The listing builds one solid part. Answer for the finished solid, in the listing's coordinates (mm). Face numbers are marked on the shaded views. A direction names the side the tool comes from. Coordinates: 2 decimals unless noted, no trailing zeros. Order: outer loops, then holes, each group sorted by start corner. A loop starts at its lowest first (then second) coordinate and runs counter-clockwise, first axis right, second up.
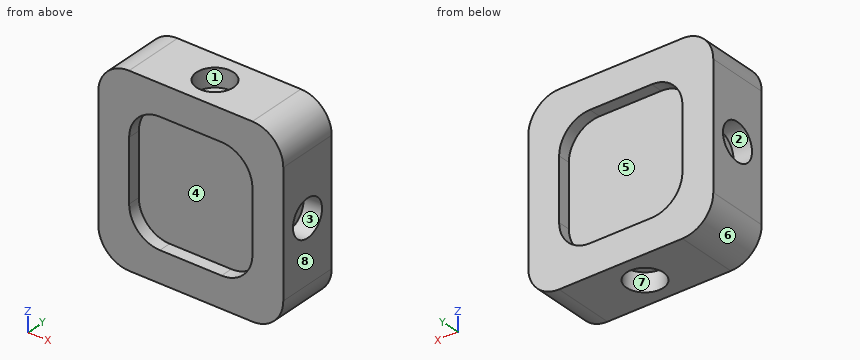
from build123d import *

# Parameters (mm, degrees)
SKETCH2_W           = 30
SKETCH2_H           = 30
BOSS_EXTRUDE1_DEPTH = 10
SKETCH3_R           = 3
CUT_EXTRUDE1_DEPTH  = 3
SKETCH4_R           = 3
CUT_EXTRUDE2_DEPTH  = 3
CUT_EXTRUDE3_START  = -3
SKETCH5_R           = 3
CUT_EXTRUDE3_DEPTH  = 3
CUT_EXTRUDE4_START  = -3
SKETCH6_R           = 3
CUT_EXTRUDE4_DEPTH  = 3
FILLET1_R           = 5
SKETCH8_W           = 20
SKETCH8_H           = 20
CUT_EXTRUDE6_DEPTH  = 2
FILLET2_R           = 5
SKETCH9_W           = 20
SKETCH9_H           = 20
CUT_EXTRUDE7_DEPTH  = 2
FILLET3_R           = 5


with BuildPart() as part:
    # Sketch2 → Boss-Extrude1 (new body)
    with BuildSketch(Plane(origin=(0, 0, 0), x_dir=(1, 0, 0), z_dir=(0, 1, 0))):
        Rectangle(SKETCH2_W, SKETCH2_H)
    extrude(amount=BOSS_EXTRUDE1_DEPTH)

    # Sketch3 → Cut-Extrude1 (cut)
    with BuildSketch(Plane.XY.offset(15)):
        with Locations((0, 5)):
            Circle(SKETCH3_R)
    extrude(amount=-CUT_EXTRUDE1_DEPTH, mode=Mode.SUBTRACT)

    # Sketch4 → Cut-Extrude2 (cut)
    with BuildSketch(Plane(origin=(15, 0, 0), x_dir=(0, 0, -1), z_dir=(1, 0, 0))):
        with Locations((0, 5)):
            Circle(SKETCH4_R)
    extrude(amount=-CUT_EXTRUDE2_DEPTH, mode=Mode.SUBTRACT)

    # Sketch5 → Cut-Extrude3 (cut)
    with BuildSketch(Plane(origin=(0, 0, -15), x_dir=(-1, 0, 0), z_dir=(0, 0, -1)).offset(CUT_EXTRUDE3_START)):
        with Locations(Location((0, 5, 0), (0, 0, 180))):
            Circle(SKETCH5_R)
    extrude(amount=CUT_EXTRUDE3_DEPTH, mode=Mode.SUBTRACT)

    # Sketch6 → Cut-Extrude4 (cut)
    with BuildSketch(Plane.ZY.offset(15).offset(CUT_EXTRUDE4_START)):
        with Locations(Location((0, 5, 0), (0, 0, 180))):
            Circle(SKETCH6_R)
    extrude(amount=CUT_EXTRUDE4_DEPTH, mode=Mode.SUBTRACT)

    # Fillet1
    fillet1_edges = [part.edges().sort_by_distance(p)[0] for p in [
        (15, 5, 15),
        (-15, 5, 15),
        (-15, 5, -15),
        (15, 5, -15),
    ]]
    fillet(fillet1_edges, radius=FILLET1_R)

    # Sketch8 → Cut-Extrude6 (cut)
    with BuildSketch(Plane(origin=(0, 10, 0), x_dir=(1, 0, 0), z_dir=(0, 1, 0))):
        Rectangle(SKETCH8_W, SKETCH8_H)
    extrude(amount=-CUT_EXTRUDE6_DEPTH, mode=Mode.SUBTRACT)

    # Fillet2
    fillet2_edges = [part.edges().sort_by_distance(p)[0] for p in [
        (10, 9, -10),
        (10, 9, 10),
        (-10, 9, 10),
        (-10, 9, -10),
    ]]
    fillet(fillet2_edges, radius=FILLET2_R)

    # Sketch9 → Cut-Extrude7 (cut)
    with BuildSketch(Plane(origin=(0, 0, 0), x_dir=(-1, 0, 0), z_dir=(0, -1, 0))):
        Rectangle(SKETCH9_W, SKETCH9_H)
    extrude(amount=-CUT_EXTRUDE7_DEPTH, mode=Mode.SUBTRACT)

    # Fillet3
    fillet3_edges = [part.edges().sort_by_distance(p)[0] for p in [
        (10, 1, 10),
        (10, 1, -10),
        (-10, 1, -10),
        (-10, 1, 10),
    ]]
    fillet(fillet3_edges, radius=FILLET3_R)


solid = part.part
1) Determine the mould class of the marked faces 5, 6, 7 and 8 for opening direction X: released by +X, released by -X, zero draft, split by the parting line, or undercut.
2) A tool of negligible diameter and unlimited length cuts with its end or side. For the marked faces 1, 2, 3 and 4, from which of +Z, -Z, +X, -X, +Y, -Y can it reach the whole face along a straight path? Write none if from no direction.
3) Section C-C (x = -5.75) is taken. Give the vertices of the cut face in (y, z), then the cut area to 3 significant figures.
4) Consider L1, parallel to Y at x = 0, z = -12.9; L2, parallel to Z at x = 0.25, y = 9; L3, parallel to Z at x = 1.5, y = 3. Determine where each line is inside the solid, lowest interval first.
5) Section D-D (x = -12.5) is taken. Give the vertices of the cut face in (y, z).
6) Section B-B (y = 5) is taken. Give the vertices of the cut face in (x, z), then the cut area to 3 significant figures.
7) Each of these flat-tipped pins is pushed along its axis until it touches: P1, Ø10, axis at x = -1.5, z = -3.5, coming from the +Y side; P2, Ø3.5, axis at x = 0, y = 5, coming from the -Z side; P3, Ø16, axis at x = 1.5, z = 1.5, coming from the -Y side. Where does it stop, or does it pass through?
8) Section A-A (z = 0) is taken. Give the vertices of the cut face in (x, y).
Filled sheet:
1. face 5: undercut
1. face 6: released by -X
1. face 7: undercut
1. face 8: released by +X
2. face 1: +Z
2. face 2: -X
2. face 3: +X
2. face 4: -Y
3. outline: (0, -15) - (10, -15) - (10, -9.94) - (8, -9.94) - (8, 9.94) - (10, 9.94) - (10, 15) - (0, 15) - (0, 9.94) - (2, 9.94) - (2, -9.94) - (0, -9.94) - close
3. area: 220 mm2
4. L1: y = 0 to 2, 8 to 10
4. L2: z = -15 to -10, 10 to 15
4. L3: z = -12 to 12
5. outline: (0, -14.33) - (10, -14.33) - (10, 14.33) - (0, 14.33) - close; hole circle Ø6 at (5, 0)
6. outline: (-15, -10) arc R5 ccw to (-10, -15) - (-3, -15) - (-3, -12) - (3, -12) - (3, -15) - (10, -15) arc R5 ccw to (15, -10) - (15, -3) - (12, -3) - (12, 3) - (15, 3) - (15, 10) arc R5 ccw to (10, 15) - (3, 15) - (3, 12) - (-3, 12) - (-3, 15) - (-10, 15) arc R5 ccw to (-15, 10) - (-15, 3) - (-12, 3) - (-12, -3) - (-15, -3) - close
6. area: 807 mm2
7. P1: stops at y = 8
7. P2: stops at z = -12
7. P3: stops at y = 2
8. outline: (-15, 0) - (-10, 0) - (-10, 2) - (10, 2) - (10, 0) - (15, 0) - (15, 2) - (12, 2) - (12, 8) - (15, 8) - (15, 10) - (10, 10) - (10, 8) - (-10, 8) - (-10, 10) - (-15, 10) - (-15, 8) - (-12, 8) - (-12, 2) - (-15, 2) - close
